from build123d import *

# Parameters (mm, degrees)
SKETCH1_W             = 10
SKETCH1_H             = 112
BOSS_EXTRUDE1_DEPTH   = 12.75
BOSS_EXTRUDE1_2_DEPTH = 12.75
FILLET1_R             = 4
FILLET2_R             = 4
SKETCH2_R             = 1.5
SKETCH2_R_2           = 3
CUT_EXTRUDE1_DEPTH    = 13.75
SKETCH3_W             = 48
SKETCH3_H             = 34
CUT_EXTRUDE2_DEPTH    = 12.75
SKETCH4_R             = 5
SKETCH4_R_2           = 4.5
CUT_EXTRUDE3_DEPTH    = 13.75
SKETCH5_W             = 10
SKETCH5_H             = 3
BOSS_EXTRUDE2_DEPTH   = 44
BOSS_EXTRUDE3_REACH   = 58
SKETCH6_W             = 10
SKETCH6_H             = 3
FILLET3_R             = 1


with BuildPart() as part:
    # Sketch1 → Boss-Extrude1 (new body)
    with BuildSketch(Plane(origin=(0, 0, 0), x_dir=(1, 0, 0), z_dir=(0, 1, 0))):
        with Locations((-27, 56)):
            Rectangle(SKETCH1_W, SKETCH1_H)
    extrude(amount=BOSS_EXTRUDE1_DEPTH)

    # Fillet2
    fillet2_edges = [part.edges().sort_by_distance(p)[0] for p in [
        (-22, 6.375, -112),
        (-22, 6.375, 0),
        (-32, 6.375, 0),
        (-32, 6.375, -112),
    ]]
    fillet(fillet2_edges, radius=FILLET2_R)


with BuildPart() as body_2:
    # Sketch1 → Boss-Extrude1 2 (new body)
    with BuildSketch(Plane(origin=(0, 0, 0), x_dir=(1, 0, 0), z_dir=(0, 1, 0))):
        with Locations((27, 56)):
            Rectangle(SKETCH1_W, SKETCH1_H)
    extrude(amount=BOSS_EXTRUDE1_2_DEPTH)

    # Fillet1
    fillet1_edges = [body_2.edges().sort_by_distance(p)[0] for p in [
        (22, 6.375, 0),
        (22, 6.375, -112),
        (32, 6.375, -112),
        (32, 6.375, 0),
    ]]
    fillet(fillet1_edges, radius=FILLET1_R)


with BuildPart() as cut_extrude1_tool:
    # Sketch2 → Cut-Extrude1 (new body, through all)
    with BuildSketch(Plane(origin=(0, 12.75, 0), x_dir=(1, 0, 0), z_dir=(0, 1, 0))):
        with Locations((-26.5, 101)):
            Circle(SKETCH2_R)
        with Locations((26.5, 101)):
            Circle(SKETCH2_R)
        with Locations((26.5, 11)):
            Circle(SKETCH2_R)
        with Locations((-26.5, 11)):
            Circle(SKETCH2_R)
        with Locations((0, 38)):
            Circle(SKETCH2_R_2)
    extrude(amount=-CUT_EXTRUDE1_DEPTH)


with BuildPart() as part_1:
    add(part.part)

    # Cut-Extrude1: cut by cut_extrude1_tool
    add(cut_extrude1_tool.part, mode=Mode.SUBTRACT)


with BuildPart() as body_2_1:
    add(body_2.part)

    # Cut-Extrude1: cut by cut_extrude1_tool
    add(cut_extrude1_tool.part, mode=Mode.SUBTRACT)


with BuildPart() as cut_extrude2_tool:
    # Sketch3 → Cut-Extrude2 (new body)
    with BuildSketch(Plane(origin=(0, 12.75, 0), x_dir=(1, 0, 0), z_dir=(0, 1, 0))):
        with Locations((0, 33)):
            Rectangle(SKETCH3_W, SKETCH3_H)
    extrude(amount=-CUT_EXTRUDE2_DEPTH)


with BuildPart() as part_2:
    add(part_1.part)

    # Cut-Extrude2: cut by cut_extrude2_tool
    add(cut_extrude2_tool.part, mode=Mode.SUBTRACT)


with BuildPart() as body_2_2:
    add(body_2_1.part)

    # Cut-Extrude2: cut by cut_extrude2_tool
    add(cut_extrude2_tool.part, mode=Mode.SUBTRACT)


with BuildPart() as cut_extrude3_tool:
    # Sketch4 → Cut-Extrude3 (new body, through all)
    with BuildSketch(Plane.XZ):
        with Locations((18.538884711, -69.4)):
            Circle(SKETCH4_R)
        with Locations((-18.538884711, -99.6)):
            Circle(SKETCH4_R)
        with Locations((-18.538884711, -6.6)):
            Circle(SKETCH4_R)
        with Locations((30.838884711, -51)):
            Circle(SKETCH4_R_2)
        with Locations((-30.838884711, -25)):
            Circle(SKETCH4_R_2)
        with BuildLine():
            ThreePointArc((31.774007787, -109.75), (30.281326332, -111.686308388), (27.856664361, -112))
            add(Edge.make_bspline(
                [(31.774007787, -109.75), (30.468226645, -110.5), (29.162445503, -111.25), (27.856664361, -112)],
                knots=[0, 0, 0, 0, 1, 1, 1, 1], degree=3))
        make_face()
    extrude(amount=-CUT_EXTRUDE3_DEPTH)


with BuildPart() as part_3:
    add(part_2.part)

    # Cut-Extrude3: cut by cut_extrude3_tool
    add(cut_extrude3_tool.part, mode=Mode.SUBTRACT)



with BuildPart() as body_2_3:
    add(body_2_2.part)

    # Cut-Extrude3: cut by cut_extrude3_tool
    add(cut_extrude3_tool.part, mode=Mode.SUBTRACT)


with BuildPart() as part_4:
    add(part_3.part)

    add(body_2_3.part)  # Boss-Extrude2 merges body 2
    # Sketch5 → Boss-Extrude2 (add)
    with BuildSketch(Plane(origin=(-22, 0, 0), x_dir=(0, 0, -1), z_dir=(1, 0, 0))):
        with Locations((85.991581932, 1.5)):
            Rectangle(SKETCH5_W, SKETCH5_H)
    extrude(amount=BOSS_EXTRUDE2_DEPTH)

    # Sketch6 → Boss-Extrude3 (add, up to next)
    with BuildSketch(Plane(origin=(-24, 0, 0), x_dir=(0, 0, -1), z_dir=(1, 0, 0)), mode=Mode.PRIVATE) as boss_extrude3_sk1:
        with Locations((39, 1.5)):
            Rectangle(SKETCH6_W, SKETCH6_H)
    boss_extrude3_tool1 = extrude(boss_extrude3_sk1.sketch, amount=BOSS_EXTRUDE3_REACH, mode=Mode.PRIVATE) - part_4.part
    add(boss_extrude3_tool1.solids().sort_by_distance((-24, 1.5, -39))[0])

    # Fillet3
    fillet3_edges = [part_4.edges().sort_by_distance(p)[0] for p in [
        (0, 3, -90.991581932),
        (0, 3, -80.991581932),
        (-22, 6.375, -50),
        (-22, 6.375, -16),
        (0, 3, -34),
        (0, 3, -44),
        (22, 6.375, -16),
        (22, 6.375, -50),
    ]]
    fillet(fillet3_edges, radius=FILLET3_R)


solid = part_4.part
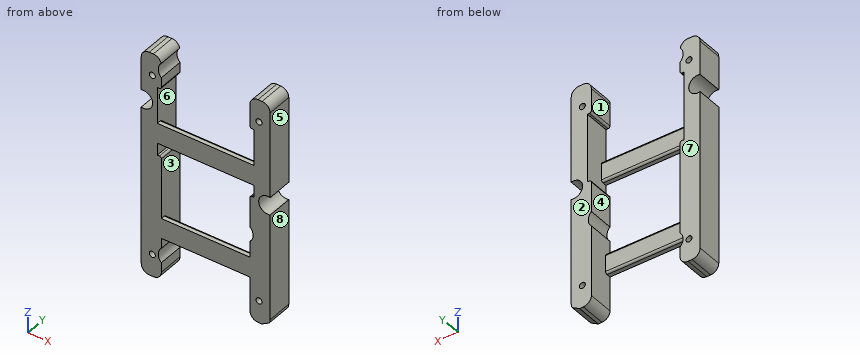
For this review, take the finished solid that the model builds, in its own axes (mm). Face numbers are marked on the shaded views. A direction names the side the tool comes from. Round coordinates to 2 decimals unless told otherwise and drop trailing zeros. Loops run counter-clockwise (first coordinate to the right, second up) from the corner with the lowest first, then second, coordinate; pieces in that order, holes last. Notation, with made-up numbers: (45, 0) - (92, 0) arc R29 cw to (92, 23) - close; hole circle Ø5 at (88, -32.5). An arc over 180 degrees is marked (long way). Use one line per item in the form item = value.
Item 1: Consider section C-C on y = 5.75. State how many separate pieces and enclosed holes the cut face has, then the cut area to 3 significant figures.
Answers:
separate_pieces = 2
enclosed_holes = 4
area = 1,940 mm^2
Item 2: Consider section D-D on z = -101. Write out the cut boundary in (x, y), then the cut area to 3 significant figures.
Answers:
outline = (-32, 0) - (-28, 0) - (-28, 12.75) - (-32, 12.75) - close; (-25, 0) - (-23.34, 0) - (-23.34, 12.75) - (-25, 12.75) - close; (22, 0) - (25, 0) - (25, 12.75) - (22, 12.75) - close; (28, 0) - (32, 0) - (32, 12.75) - (28, 12.75) - close
area = 161 mm^2
Item 3: Clearance check with flat-ended pins moving along their axes: P1, Ø1, axis at x = 17, y = 2.5, coming from the -Z side; P2, Ø3, axis at x = -8, y = 4, coming from the +Z side; P3, Ø1.1, axis at x = -23.5, y = 5.5, coming from the +Z side. State where each tip first meets the part, or that it passes through.
Answers:
P1 = -90.99
P2 = -34.13
P3 = -0.51
Item 4: Consider section A-A on x = -15.5. Write out the cut boundary in (y, z).
Answers:
outline = (0, -90.99) - (2, -90.99) arc R1 ccw to (3, -89.99) - (3, -81.99) arc R1 ccw to (2, -80.99) - (0, -80.99) - close; (0, -44) - (2, -44) arc R1 ccw to (3, -43) - (3, -35) arc R1 ccw to (2, -34) - (0, -34) - close
Item 5: Tool access review of the marked faces 1, 2, 3, 4 and 5: name each direction out of +Z, -Z, +X, -X, +Y, -Y from which nothing blocks a thin tool from reaching the whole face with its end or side.
Answers:
face_1 = +Z, +Y, -Y
face_2 = +Z, -Z, +X, -X, +Y
face_3 = +Y
face_4 = +Y, -Y
face_5 = +Z, -Z, +X, +Y, -Y
Item 6: Consider section B-B on z = -25. Write out the cut boundary in (x, y), then the cut area to 3 significant figures.
Answers:
outline = (-26.34, 0) - (-24, 0) - (-24, 12.75) - (-26.34, 12.75) - close; (24, 0) - (32, 0) - (32, 12.75) - (24, 12.75) - close
area = 132 mm^2
Item 7: For line 1 (X direction, y = 6.25, z = -25); line 2 (X direction, y = 9.5, z = -101); line 3 (Z direction, x = 23, y = 10.5), list the stretches that pass through material, from the lowest coordinate up.
Answers:
line_1 = -26.34 to -24, 24 to 32
line_2 = -32 to -28, -25 to -23.34, 22 to 25, 28 to 32
line_3 = -110.65 to -71.66, -67.14 to -50, -16 to -1.35
Item 8: Mouldability with a two-part tool opening along X and no side actions: class the marked faces 6, 7 and 8 as +X half, -X half, draft (parallel to the pull), parting line (faces both ways), or undercut.
Answers:
face_6 = undercut
face_7 = draft
face_8 = +X half
